```python
from build123d import *

# Parameters (mm, degrees)
SKETCH_W        = 250
SKETCH_H        = 46
PAD_DEPTH       = 60
SKETCH001_R     = 8
SKETCH001_R_2   = 6
POCKET_DEPTH    = 60.001
SKETCH002_W     = 95
SKETCH002_H     = 40
POCKET001_DEPTH = 40
SKETCH003_R     = 11.05
POCKET002_DEPTH = 7


with BuildPart() as part:
    # Sketch → Pad (new body)
    with BuildSketch(Plane.XZ):
        with Locations((0, -1.847977)):
            Rectangle(SKETCH_W, SKETCH_H)
    extrude(amount=-PAD_DEPTH)

    # Sketch001 → Pocket (cut, through all)
    with BuildSketch(Plane.XZ):
        with Locations((-79, 0)):
            Circle(SKETCH001_R)
        Circle(SKETCH001_R_2)
        with Locations((79, 0)):
            Circle(SKETCH001_R)
    extrude(amount=-POCKET_DEPTH, mode=Mode.SUBTRACT)

    # Sketch002 → Pocket001 (cut)
    with BuildSketch(Plane(origin=(0, 0, 21.152023), x_dir=(-1, 0, 0), z_dir=(0, 0, 1))):
        with Locations((-67.5, -30)):
            Rectangle(SKETCH002_W, SKETCH002_H)
        with Locations((67.5, -30)):
            Rectangle(SKETCH002_W, SKETCH002_H)
    extrude(amount=-POCKET001_DEPTH, mode=Mode.SUBTRACT)

    # Sketch003 → Pocket002 (cut)
    with BuildSketch(Plane.XZ):
        Circle(SKETCH003_R)
    extrude(amount=-POCKET002_DEPTH, mode=Mode.SUBTRACT)


solid = part.part
```
Read the model definition and answer for the solid it produces. Units are mm, in the model's axes. A direction names the side the tool comes from. Coordinates: 2 decimals unless noted, no trailing zeros. Loops run counter-clockwise (first coordinate to the right, second up) from the corner with the lowest first, then second, coordinate; pieces in that order, holes last. Notation, with made-up numbers: (33, -4) -> (81, -4) arc R19 ccw to (81, 6) -> close; hole circle Ø5 at (79.25, 15.5). An arc over 180 degrees is marked (long way). Return JSON: item names as keys, results as strings.
Item 1: Flat-ended cylindrical pins translate along their axes: P1, Ø7, axis at x = 0, z = 0, coming from the +Y side; P2, Ø20, axis at x = 0, z = 0, coming from the -Y side; P3, Ø4, axis at x = 8, z = 14, coming from the -Y side; P4, Ø10, axis at x = 39.5, y = 37, coming from the +Z side. Find the tip coordinate at first contact, or state that the pin passes through.
Answers:
{"P1": "passes through", "P2": "stops at y = 7", "P3": "stops at y = 0", "P4": "stops at z = -18.85"}
Item 2: For a pull along Z with two mould halves and no side action, classify faces 1 (the flat face through (-2, 30, -24.848)), 2 (the cylindrical face through (72.651, 54.93, -4.868)), 3 (the flat face through (-67, 30, -18.848)), 4 (the flat face through (125, 30, -2)) as +Z half, -Z half, draft (parallel to the pull), parting line (faces both ways), or undercut.
Answers:
{"face 1": "-Z half", "face 2": "undercut", "face 3": "+Z half", "face 4": "draft"}
Item 3: For faces 5 (the flat face through (5, 7, -5)), 6 (the flat face through (-2, 60, -7)), 7 (the flat face through (-115, 30, 1)), determine the directions among +Z, -Z, +X, -X, +Y, -Y from which every point of the face is accessible in a straight line to the end or side of a thin tool.
Answers:
{"face 5": "-Y", "face 6": "+Z, -Z, +X, -X, +Y", "face 7": "+Z"}
Item 4: Find section A-A (x = -79). Determine the outline of the cut face in (y, z), plus the area to 3 significant figures.
Answers:
{"outline": "(0, -24.85) -> (60, -24.85) -> (60, -8) -> (50, -8) -> (50, -18.85) -> (10, -18.85) -> (10, -8) -> (0, -8) -> close; (0, 8) -> (10, 8) -> (10, 21.15) -> (0, 21.15) -> close; (50, 8) -> (60, 8) -> (60, 21.15) -> (50, 21.15) -> close", "area": "840 mm2"}
Item 5: Find the intervals of material crossed by probe 1 along X at (y, z) = (28, -15); probe 2 along X at (y, z) = (27, 0.5); probe 3 along Y at (x, z) = (-37, -3), in increasing order.
Answers:
{"probe 1": "x = -125 to -115, -20 to 20, 115 to 125", "probe 2": "x = -125 to -115, -20 to -5.98, 5.98 to 20, 115 to 125", "probe 3": "y = 0 to 10, 50 to 60"}
Item 6: Find section B-B (x = 0). Determine the outline of the cut face in (y, z).
Answers:
{"outline": "(0, -24.85) -> (60, -24.85) -> (60, -6) -> (7, -6) -> (7, -11.05) -> (0, -11.05) -> close; (0, 11.05) -> (7, 11.05) -> (7, 6) -> (60, 6) -> (60, 21.15) -> (0, 21.15) -> close"}
Item 7: Find section C-C (y = 43). Determine the outline of the cut face in (x, z).
Answers:
{"outline": "(-125, -24.85) -> (125, -24.85) -> (125, 21.15) -> (115, 21.15) -> (115, -18.85) -> (20, -18.85) -> (20, 21.15) -> (-20, 21.15) -> (-20, -18.85) -> (-115, -18.85) -> (-115, 21.15) -> (-125, 21.15) -> close; hole circle Ø12 at (0, 0)"}
Item 8: Find section D-D (z = -15). Determine the outline of the cut face in (x, y).
Answers:
{"outline": "(-125, 0) -> (125, 0) -> (125, 60) -> (-125, 60) -> close; hole (-115, 10) -> (-20, 10) -> (-20, 50) -> (-115, 50) -> close; hole (20, 10) -> (115, 10) -> (115, 50) -> (20, 50) -> close"}
